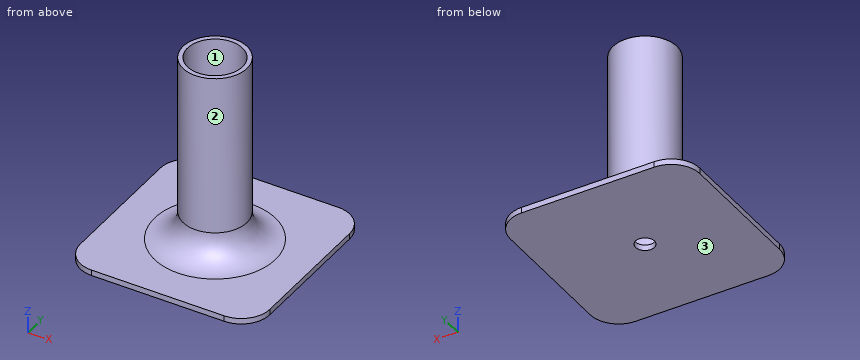
```python
from build123d import *

# Parameters (mm, degrees)
F0_W     = 100
F0_H     = 100
F1_DEPTH = 3
F2_R     = 16.9
F2_R_2   = 14.5
F3_DEPTH = 100
F4_R     = 15
F5_R     = 5
F6_DEPTH = 25


with BuildPart() as f1:
    # F0 (on Top) → F1 (new body)
    with BuildSketch(Plane.XY):
        Rectangle(F0_W, F0_H)
    extrude(amount=F1_DEPTH)

    # F2 (on face) → F3 (join)
    with BuildSketch(Plane.XY.offset(3)):
        Circle(F2_R)
        Circle(F2_R_2, mode=Mode.SUBTRACT)
    extrude(amount=F3_DEPTH)

    # F4
    f4_edges = [f1.edges().sort_by_distance(p)[0] for p in [
        (-16.9, 0, 3),
        (50, -50, 1.5),
        (50, 50, 1.5),
        (-50, 50, 1.5),
        (-50, -50, 1.5),
    ]]
    fillet(f4_edges, radius=F4_R)

    # F5 (on face) → F6 (cut)
    with BuildSketch(Plane.XY.offset(3)):
        Circle(F5_R)
    extrude(amount=-F6_DEPTH, mode=Mode.SUBTRACT)


solid = f1.part
```
Build history of the part. All positions in model axes, mm. Face numbers are marked on the shaded views. Give positions to 0.01 mm unless a question says otherwise; leave off trailing zeros. Loops run counter-clockwise (first coordinate to the right, second up) from the corner with the lowest first, then second, coordinate; pieces in that order, holes last. Notation, with made-up numbers: (4, 44) - (8, 44) arc R12 ccw to (8, 58) - close; hole circle Ø9 at (-30.75, 47.25). An arc over 180 degrees is marked (long way). Use a Markdown table: item, result.
(1) Band-saw the part on A-A (x = 0). Give the cut face in (y, z), and give its area (3 significant figures).
Taken from the geometry:
| item | result |
|---|---|
| outline | (-50, 0) - (-5, 0) - (-5, 3) - (-14.5, 3) - (-14.5, 103) - (-16.9, 103) - (-16.9, 18) arc R15 cw to (-31.9, 3) - (-50, 3) - close; (5, 0) - (50, 0) - (50, 3) - (31.9, 3) arc R15 cw to (16.9, 18) - (16.9, 103) - (14.5, 103) - (14.5, 3) - (5, 3) - close |
| area | 847 mm2 |
(2) Band-saw the part on D-D (y = -39). Give the cut face in (x, z), and give its area (3 significant figures).
Taken from the geometry:
| item | result |
|---|---|
| outline | (-49.46, 0) - (49.46, 0) - (49.46, 3) - (-49.46, 3) - close |
| area | 297 mm2 |
(3) Band-saw the part on C-C (z = 92.5). Give the cut face in (x, y).
Taken from the geometry:
| item | result |
|---|---|
| outline | circle Ø33.8 at (0, 0); hole circle Ø29 at (0, 0) |
(4) Drop flat-ended pins along their axis: pin 1 Ø3 at (x, z) = (4.5, 29) entering from -Y; pin 2 Ø1.5 at (x, y) = (-32.5, -1.5) entering from -Z; pin 3 Ø12 at (x, z) = (-10, 79) entering from -Y; pin 4 Ø6 at (x, z) = (-15.5, 29) entering from -Y. Give the stop position or say it passes through.
Taken from the geometry:
| item | result |
|---|---|
| pin 1 | y = -16.63 |
| pin 2 | z = 0 |
| pin 3 | y = -16.42 |
| pin 4 | y = -11.37 |
(5) Wall check: line 1 along Y through (x, z) = (0, 77.5); line 2 along Y through (x, z) = (0, 1); line 3 along Z through (x, y) = (31, -45.5). Give the ranges that are in metal, low to high.
Taken from the geometry:
| item | result |
|---|---|
| line 1 | -16.9 to -14.5, 14.5 to 16.9 |
| line 2 | -50 to -5, 5 to 50 |
| line 3 | 0 to 3 |
(6) Pull direction Y, two halves, no side cores. Call the marked faces 1, 2 and 3: +Y half, -Y half, draft (parallel to the pull), parting line (faces both ways), or undercut.
Taken from the geometry:
| item | result |
|---|---|
| face 1 | undercut |
| face 2 | parting line |
| face 3 | draft |
